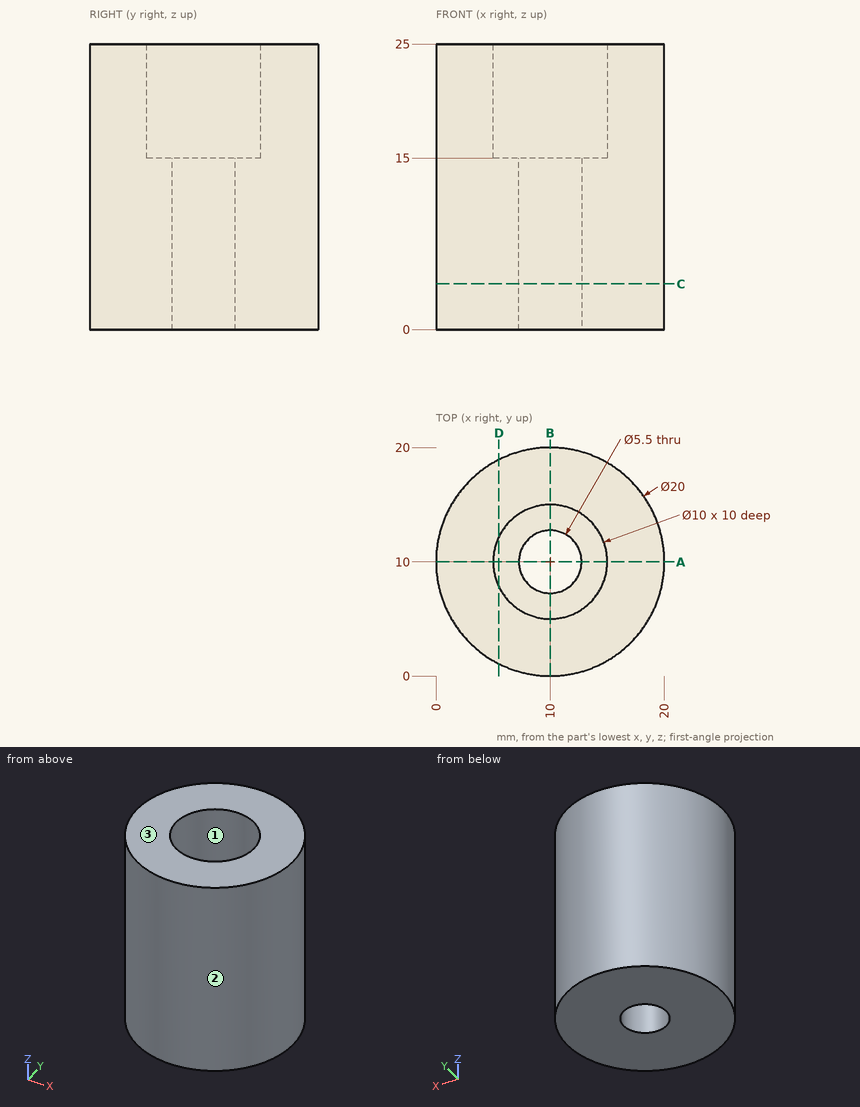
Study the drawing (mm; zero at the part's minimum x, y, z) and answer. Give positions to 0.01 mm unless a question says otherwise; leave off trailing zeros. Loops run counter-clockwise (first coordinate to the right, second up) from the corner with the lowest first, then second, coordinate; pieces in that order, holes last. Notation, with made-up numbers: M 71.5,74.25 L 75.5,74.25 A20 ccw 75.5,112.25 Z; hole C 6,50 d3. An arc over 180 degrees is marked long. Answer as CSV lines item,"result".
Item 1: Straight lines are drawn through the part: line 1 along Y through (x, z) = (10, 21); line 2 along Y through (x, z) = (10, 12); line 3 along Z through (x, y) = (6.5, 6.5). For each, find the intervals that lie inside material, in ascending order. Write a range as [from, to].
Values follow:
line 1,"y = [0, 5], [15, 20]"
line 2,"y = [0, 7.25], [12.75, 20]"
line 3,"z = [0, 15]"
Item 2: Given pin 1 Ø1.5 at (x, y) = (14.5, 10.5) entering from +Z; pin 2 Ø3 at (x, y) = (10.5, 11) entering from +Z; pin 3 Ø4 at (y, z) = (2.5, 6) entering from +X; pin 4 Ø10 at (y, z) = (17, 22) entering from -X, each flat-ended and moving along its own axis, determine where each tip first touches the part or whether it passes through.
Values follow:
pin 1,"stops at z = 25"
pin 2,"passes through"
pin 3,"stops at x = 18.35"
pin 4,"stops at x = 0.2"
Item 3: The part is cut by section A-A (y = 10). Give the vertices of the cut face in (x, z).
Values follow:
outline,"M 0,0 L 7.25,0 L 7.25,15 L 5,15 L 5,25 L 0,25 Z; M 12.75,0 L 20,0 L 20,25 L 15,25 L 15,15 L 12.75,15 Z"
Item 4: The part is cut by section C-C (z = 4). Give the vertices of the cut face in (x, y), and give its area (3 significant figures).
Values follow:
outline,"C 10,10 d20; hole C 10,10 d5.5"
area,"290 mm^2"
Item 5: The mould has two halves that part along X. Classify the marked faces 1, 2 and 3: released by +X, released by -X, zero draft, split by the parting line, or undercut.
Values follow:
face 1,"undercut"
face 2,"split by the parting line"
face 3,"zero draft"
Item 6: The part is cut by section D-D (x = 5.5). Give the vertices of the cut face in (y, z), and give its area (3 significant figures).
Values follow:
outline,"M 1.07,0 L 18.93,0 L 18.93,25 L 12.18,25 L 12.18,15 L 7.82,15 L 7.82,25 L 1.07,25 Z"
area,"403 mm^2"
